from build123d import *

# Parameters (mm, degrees)
SKETCH1_W                   = 64
SKETCH1_H                   = 62
SKETCH1_R                   = 2.5
SKETCH1_R_2                 = 3
BOSS_EXTRUDE1_DEPTH         = 6
CUT_EXTRUDE1_REACH          = 8
CUT_EXTRUDE2_REACH          = 8
FILLET1_R                   = 3
FILLET2_R                   = 3
TAP_DRILL_FOR_M3_TAP1_D     = 2.5
TAP_DRILL_FOR_M3_TAP1_DEPTH = 9
TAP_DRILL_FOR_M3_TAP1_TIP   = 0.751075774
CUT_EXTRUDE3_DEPTH          = 3
CUT_EXTRUDE4_REACH          = 5
SKETCH10_R                  = 1.5
SKETCH11_R                  = 2.5
CUT_EXTRUDE5_DEPTH          = 6
LPATTERN1_COUNT             = 3
LPATTERN1_PITCH             = 4
FILLET3_R                   = 1
SKETCH12_W                  = 22.982575198
SKETCH12_H                  = 6
CUT_EXTRUDE6_DEPTH          = 1


with BuildPart() as part:
    # Sketch1 → Boss-Extrude1 (new body)
    with BuildSketch(Plane(origin=(0, 0, 0), x_dir=(0, 0, -1), z_dir=(1, 0, 0))):
        with Locations((32, 31)):
            Rectangle(SKETCH1_W, SKETCH1_H)
        with Locations((6, 14.5)):
            Circle(SKETCH1_R, mode=Mode.SUBTRACT)
        with Locations((50, 44)):
            Circle(SKETCH1_R_2, mode=Mode.SUBTRACT)
    extrude(amount=BOSS_EXTRUDE1_DEPTH)

    # Sketch2 → Cut-Extrude1 (cut, up to next)
    with BuildSketch(Plane(origin=(6, 0, 0), x_dir=(0, 0, -1), z_dir=(1, 0, 0)), mode=Mode.PRIVATE) as cut_extrude1_sk1:
        with BuildLine():
            Line((7.732242893, 20.244504727), (27.593137265, 14.255495273))
            ThreePointArc((27.593137265, 14.255495273), (32.470162023, 14.890171527), (35.234226676, 18.958110934))
            Line((35.234226676, 18.958110934), (43, 63))
            Line((43, 63), (0, 63))
            Line((0, 63), (0, 14.5))
            ThreePointArc((0, 14.5), (2.421834084, 19.316298234), (7.732242893, 20.244504727))
        make_face()
    cut_extrude1_tool1 = extrude(cut_extrude1_sk1.sketch, amount=-CUT_EXTRUDE1_REACH, mode=Mode.PRIVATE) & part.part
    add(cut_extrude1_tool1.solids().sort_by_distance((6, 40.863189, -19.912877))[0], mode=Mode.SUBTRACT)

    # Sketch3 → Cut-Extrude2 (cut, up to next)
    with BuildSketch(Plane(origin=(6, 0, 0), x_dir=(0, 0, -1), z_dir=(1, 0, 0)), mode=Mode.PRIVATE) as cut_extrude2_sk1:
        Polygon((64, 0), (52, 0), (54.225932994, 25.442530542), (64, 29), align=None)
    cut_extrude2_tool1 = extrude(cut_extrude2_sk1.sketch, amount=-CUT_EXTRUDE2_REACH, mode=Mode.PRIVATE) & part.part
    add(cut_extrude2_tool1.solids().sort_by_distance((6, 13.1347, -58.667711))[0], mode=Mode.SUBTRACT)

    # Fillet1
    fillet1_edges = [part.edges().sort_by_distance(p)[0] for p in [
        (3, 62, -42.823673019),
    ]]
    fillet(fillet1_edges, radius=FILLET1_R)

    # Fillet2
    fillet2_edges = [part.edges().sort_by_distance(p)[0] for p in [
        (3, 25.442530542, -54.225932994),
    ]]
    fillet(fillet2_edges, radius=FILLET2_R)

    # Tap Drill for M3 Tap1
    with Locations(Plane(origin=(0, 0, 0), x_dir=(-1, 0, 0), z_dir=(0, -1, 0))):
        with Locations((-3, 48), (-3, 12)):
            Hole(TAP_DRILL_FOR_M3_TAP1_D / 2, depth=TAP_DRILL_FOR_M3_TAP1_DEPTH)
            with Locations((0, 0, -(TAP_DRILL_FOR_M3_TAP1_DEPTH + TAP_DRILL_FOR_M3_TAP1_TIP / 2))):  # 118° drill point
                Cone(0, TAP_DRILL_FOR_M3_TAP1_D / 2, TAP_DRILL_FOR_M3_TAP1_TIP, mode=Mode.SUBTRACT)

    # Sketch9 → Cut-Extrude3 (cut)
    with BuildSketch(Plane.ZY):
        Polygon((-64, 62), (-64, 35), (-54, 35), (-37.272527114, 30.517887149), (-42.823673019, 62), align=None)
    extrude(amount=-CUT_EXTRUDE3_DEPTH, mode=Mode.SUBTRACT)

    # Sketch10 → Cut-Extrude4 (cut, up to next)
    with BuildSketch(Plane.ZY.offset(-3), mode=Mode.PRIVATE) as cut_extrude4_sk1:
        with Locations((-61, 59)):
            Circle(SKETCH10_R)
    cut_extrude4_tool1 = extrude(cut_extrude4_sk1.sketch, amount=-CUT_EXTRUDE4_REACH, mode=Mode.PRIVATE) & part.part
    add(cut_extrude4_tool1.solids().sort_by_distance((3, 59, -61))[0], mode=Mode.SUBTRACT)
    # Sketch10 → Cut-Extrude4 (cut, up to next)
    with BuildSketch(Plane.ZY.offset(-3), mode=Mode.PRIVATE) as cut_extrude4_sk2:
        with Locations((-51, 59)):
            Circle(SKETCH10_R)
    cut_extrude4_tool2 = extrude(cut_extrude4_sk2.sketch, amount=-CUT_EXTRUDE4_REACH, mode=Mode.PRIVATE) & part.part
    add(cut_extrude4_tool2.solids().sort_by_distance((3, 59, -51))[0], mode=Mode.SUBTRACT)

    # Sketch11 → Cut-Extrude5 (cut)
    with BuildSketch(Plane.ZY):
        with Locations((-9.829669818, 13.345171405)):
            Circle(SKETCH11_R)
    cut_extrude5 = extrude(amount=-CUT_EXTRUDE5_DEPTH, mode=Mode.SUBTRACT)

    # LPattern1: Cut-Extrude5 ×3
    with Locations(*[Vector(0, -0.288707149, -0.957417455) * (i * LPATTERN1_PITCH) for i in range(1, LPATTERN1_COUNT)]):
        add(cut_extrude5, mode=Mode.SUBTRACT)

    # Fillet3
    fillet3_edges = [part.edges().sort_by_distance(p)[0] for p in [
        (3, 15.358711884, -8.347895632),
        (3, 12.486459521, -7.481774186),
        (3, 14.203883289, -12.17756545),
        (3, 11.331630925, -11.311444004),
        (3, 10.17680233, -15.141113822),
        (3, 13.049054694, -16.007235268),
    ]]
    fillet(fillet3_edges, radius=FILLET3_R)

    # Sketch12 → Cut-Extrude6 (cut)
    with BuildSketch(Plane.ZY.offset(-3)):
        with Locations((-52.508712401, 59)):
            Rectangle(SKETCH12_W, SKETCH12_H)
    extrude(amount=-CUT_EXTRUDE6_DEPTH, mode=Mode.SUBTRACT)


solid = part.part
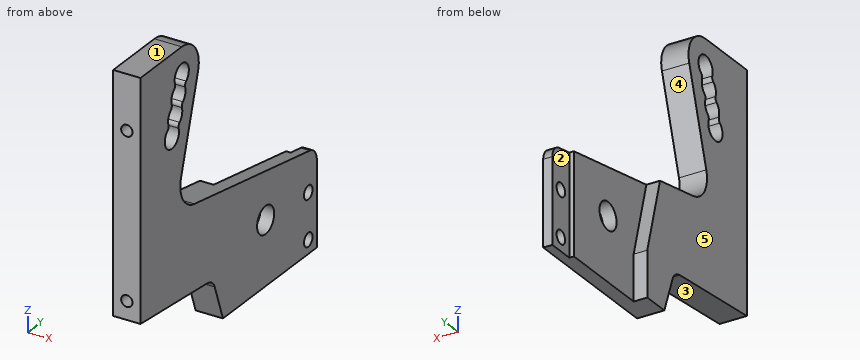
For this review, take the finished solid that the model builds, in its own axes (mm). Face numbers are marked on the shaded views. A direction names the side the tool comes from. Give positions to 0.01 mm unless a question says otherwise; leave off trailing zeros. Order: outer loops, then holes, each group sorted by start corner. A loop starts at its lowest first (then second) coordinate and runs counter-clockwise, first axis right, second up. Notation, with made-up numbers: (-23.75, 26) - (-13.75, 26) arc R18 cw to (-13.75, 55) - close; hole circle Ø2 at (-13, 3.25). An arc over 180 degrees is marked (long way). Answer as a JSON object with one key per item and string values. Group by question number.
Item 1: Take a section at D-D on z = -25. Give the boundary of the cut face in (x, y), and give its area (3 significant figures).
Item 2: Take a section at C-C on y = 39. Give the boundary of the cut face in (x, z).
Item 3: Wall thickness on line 1 along Y through (x, z) = (5.2, -50); line 2 along Y through (x, z) = (2, -6); line 3 along Z through (x, y) = (3, 2): over which ranges is each line inside the solid? List them lowest first.
Item 4: Machinability: for the marked faces 1 and 2, which of the approach directions +Z, -Z, +X, -X, +Y, -Y give a long, thin tool a straight path to every point of the face, cutting with its end or side? Answer none if there is none.
Item 5: Take a section at A-A on z = -61. Give the boundary of the cut face in (x, y), and give its area (3 significant figures).
Item 6: Draft analysis for pull direction Z (two halves, no side actions). For the marked faces 3, 4 and 5, state which applies: pulls with the +Z half, pulls with the -Z half, needs draft (parallel to the pull), parting line crosses it, or undercut.
Item 7: Take a section at B-B on z = -51. Give the boundary of the cut face in (x, y), and give its area (3 significant figures).
Item 8: Clearance check with flat-ended pins moving along their axes: pin 1 Ø2 at (x, z) = (3, -12) entering from -Y; pin 2 Ø3 at (y, z) = (14.5, -6) entering from +X; pin 3 Ø5 at (y, z) = (58, -56) entering from -X; pin 4 Ø1.5 at (x, z) = (1, -15) entering from +Y. State where each tip first meets the part, or that it passes through.
Reported:
{
 "1": {"outline": "(0, 0) - (6, 0) - (6, 15.04) - (0, 15.04) - close", "area": "90.2 mm^2"},
 "2": {"outline": "(3, -64) - (6, -64) - (6, -38.77) - (3, -38.77) - close"},
 "3": {"line 1": "0 to 41, 47 to 57.88, 60.12 to 62", "line 2": "0 to 12, 17 to 20.5", "line 3": "-52.17 to -49.25, -46.75 to -13.25, -10.75 to 0"},
 "4": {"face 1": "+Z, +X, -X, +Y, -Y", "face 2": "+Z, -Z, -X, +Y"},
 "5": {"outline": "(0, 27.91) - (6, 27.91) - (6, 57.5) - (4, 57.5) - (4, 56) - (3, 56) - (3, 35) - (0, 35) - close; (4, 60.5) - (6, 60.5) - (6, 62) - (4, 62) - close", "area": "112 mm^2"},
 "6": {"face 3": "pulls with the -Z half", "face 4": "undercut", "face 5": "needs draft"},
 "7": {"outline": "(0, 0) - (6, 0) - (6, 41.17) - (3, 41.17) - (3, 34.2) - (0, 34.2) - close; (3, 46.83) - (6, 46.83) - (6, 57.5) - (4, 57.5) - (4, 56) - (3, 56) - close; (4, 60.5) - (6, 60.5) - (6, 62) - (4, 62) - close", "area": "260 mm^2"},
 "8": {"pin 1": "y = 9.15", "pin 2": "through", "pin 3": "x = 3", "pin 4": "y = 18.28"}
}
